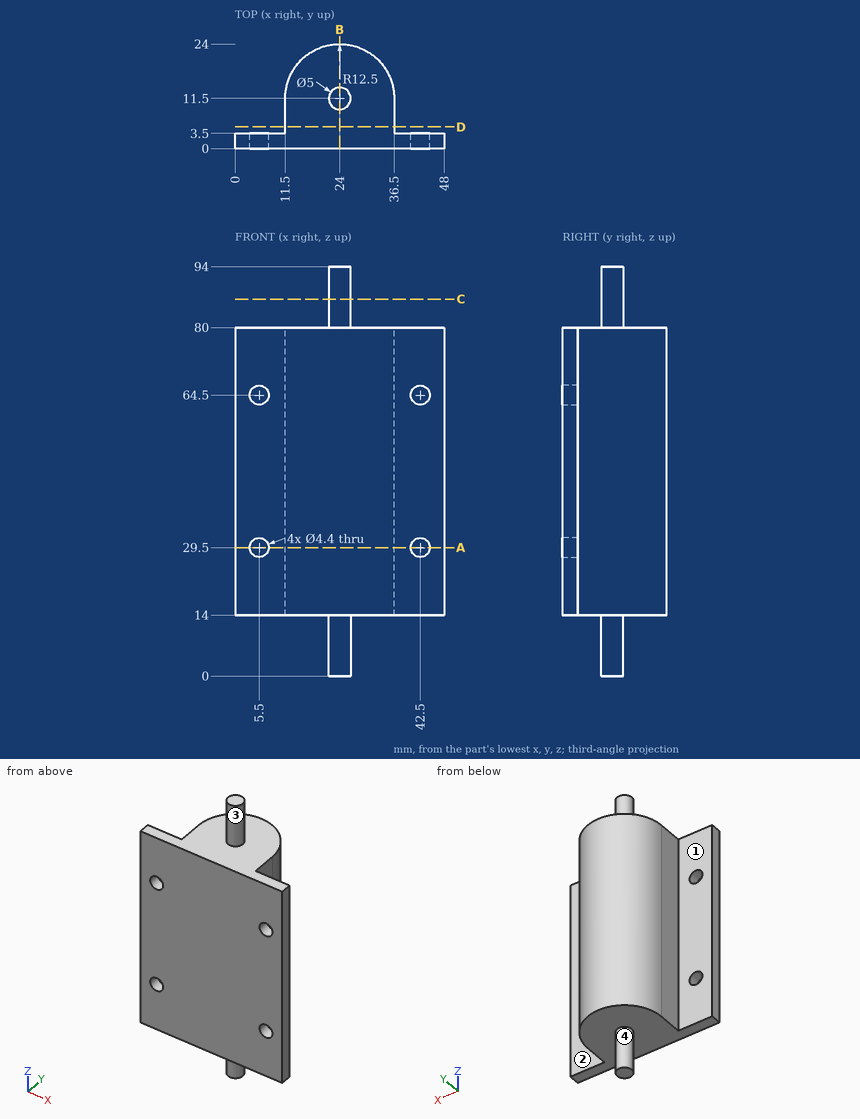
The figure shows three views and two pictorial views of one solid part (mm, origin at its lowest corner). Answer the questions. A direction names the side the tool comes from. Give positions to 0.01 mm unless a question says otherwise; leave off trailing zeros. Write each loop counter-clockwise with the first axis right and the second up, starting at its lowest first coordinate (ties: lowest second). Pieces come first, ordered by that corner, then holes. Notation, with made-up numbers: (-9.5, 11) - (15.5, 11) arc R34 cw to (15.5, 46) - close; hole circle Ø1 at (33, 49). An arc over 180 degrees is marked (long way). Use one line per item in the form item = value. Start each with the question number.
1) Find section B-B on x = 24. Determine the outline of the cut face in (y, z).
2) Find section A-A on z = 29.5. Determine the outline of the cut face in (x, y), plus the area to 3 significant figures.
3) Flat-ended cylindrical pins translate along their axes: pin 1 Ø6 at (x, z) = (11, 63.5) entering from +Y; pin 2 Ø6.5 at (y, z) = (8.5, 62) entering from +X; pin 3 Ø2.5 at (y, z) = (8, 58) entering from -X; pin 4 Ø2.5 at (x, z) = (5.5, 64.5) entering from -Y. Find the tip coordinate at first contact, or state that the pin passes through.
4) Find section D-D on y = 5. Determine the outline of the cut face in (x, z).
5) A tool of negligible diameter and unlimited length cuts with its end or side. For the marked faces 1, 2, 3 and 4, from which of +Z, -Z, +X, -X, +Y, -Y can it reach the whole face along a straight path? Write none if from no direction.
6) Find section C-C on z = 86.5. Determine the outline of the cut face in (x, y), plus the area to 3 significant figures.
7) Consider line 1 along X through (y, z) = (2.75, 29.5); line 2 along X through (y, z) = (10.5, 52); line 3 along Z through (x, y) = (19, 7.5). Determine where each line is inside the solid, lowest interval first. Write a range as from..to.
Geometry results:
q1.outline = (0, 14) - (9, 14) - (9, 0) - (14, 0) - (14, 14) - (24, 14) - (24, 80) - (14, 80) - (14, 94) - (9, 94) - (9, 80) - (0, 80) - close
q2.outline = (0, 0) - (3.3, 0) - (3.3, 3.5) - (0, 3.5) - close; (7.7, 0) - (40.3, 0) - (40.3, 3.5) - (36.5, 3.5) - (36.5, 11.5) arc R12.5 ccw to (11.5, 11.5) - (11.5, 3.5) - (7.7, 3.5) - close; (44.7, 0) - (48, 0) - (48, 3.5) - (44.7, 3.5) - close
q2.area = 583 mm2
q3.pin_1 = 19
q3.pin_2 = 36.5
q3.pin_3 = 11.5
q3.pin_4 = through
q4.outline = (11.5, 14) - (36.5, 14) - (36.5, 80) - (11.5, 80) - close
q5.face_1 = +Z, -Z, -X, +Y
q5.face_2 = +Z, -Z, +X, +Y
q5.face_3 = +Z
q5.face_4 = -Z
q6.outline = circle Ø5 at (24, 11.5)
q6.area = 19.6 mm2
q7.line_1 = 0..3.3, 7.7..40.3, 44.7..48
q7.line_2 = 11.5..36.5
q7.line_3 = 14..80
